The listing builds one solid part. Answer for the finished solid, in the listing's coordinates (mm). Face numbers are marked on the shaded views. A direction names the side the tool comes from. Give positions to 0.01 mm unless a question says otherwise; leave off trailing zeros. Order: outer loops, then holes, each group sorted by start corner. A loop starts at its lowest first (then second) coordinate and runs counter-clockwise, first axis right, second up. Notation, with made-up numbers: (-13, 24) -> (28, 24) arc R22 ccw to (28, 37) -> close; hole circle Ø4 at (57.25, -11). An arc over 180 degrees is marked (long way). Write item = value, one per line. Start each with the question number.
```python
from build123d import *

# Parameters (mm, degrees)
F0_W      = 1219.2
F0_H      = 190.5
F0_W_2    = 1181.1
F0_H_2    = 152.4
F1_DEPTH  = 762
F2_W      = 1219.2
F2_H      = 190.5
F2_W_2    = 1181.1
F2_H_2    = 152.4
F3_DEPTH  = 762
F4_W      = 1219.2
F4_H      = 622.3
F4_W_2    = 1181.1
F4_H_2    = 584.2
F5_DEPTH  = 762
F6_W      = 1219.2
F6_H      = 622.3
F6_W_2    = 1181.1
F6_H_2    = 584.2
F7_DEPTH  = 762
F8_W      = 2438.4
F8_H      = 127
F9_DEPTH  = 6.35
F10_W     = 2438.4
F10_H     = 812.8
F11_DEPTH = 19.05
F12_R     = 38.1
F13_DEPTH = 152.4
F14_W     = 19.05
F14_H     = 152.4
F15_DEPTH = 762
F17_W     = 121.444046
F17_H     = 6.35
F18_DEPTH = 2438.4


with BuildPart() as f1:
    # F0 (on Front) → F1 (new body)
    with BuildSketch(Plane.XZ):
        with Locations((-609.6, 95.25)):
            Rectangle(F0_W, F0_H)
        with Locations((-609.6, 95.25)):
            Rectangle(F0_W_2, F0_H_2, mode=Mode.SUBTRACT)
    extrude(amount=F1_DEPTH)

    # F2 (on Front) → F3 (join)
    with BuildSketch(Plane.XZ):
        with Locations((609.6, 95.25)):
            Rectangle(F2_W, F2_H)
        with Locations((609.6, 95.25)):
            Rectangle(F2_W_2, F2_H_2, mode=Mode.SUBTRACT)
    extrude(amount=F3_DEPTH)

    # F4 (on Front) → F5 (join)
    with BuildSketch(Plane.XZ):
        with Locations((-609.6, -311.15)):
            Rectangle(F4_W, F4_H)
        with Locations((-609.6, -311.15)):
            Rectangle(F4_W_2, F4_H_2, mode=Mode.SUBTRACT)
    extrude(amount=F5_DEPTH)

    # F6 (on Front) → F7 (join)
    with BuildSketch(Plane.XZ):
        with Locations((609.6, -311.15)):
            Rectangle(F6_W, F6_H)
        with Locations((609.6, -311.15)):
            Rectangle(F6_W_2, F6_H_2, mode=Mode.SUBTRACT)
    extrude(amount=F7_DEPTH)

    # F8 (on face) → F9 (cut)
    with BuildSketch(Plane.XY.offset(190.5)):
        with Locations((0, -622.3)):
            Rectangle(F8_W, F8_H)
    extrude(amount=-F9_DEPTH, mode=Mode.SUBTRACT)

    # F10 (on face) → F11 (join)
    with BuildSketch(Plane.XZ.offset(762)):
        with Locations((0, -215.9)):
            Rectangle(F10_W, F10_H)
    extrude(amount=F11_DEPTH)

    # F12 (on face) → F13 (join)
    with BuildSketch(Plane(origin=(0, 0, -622.3), x_dir=(1, 0, 0), z_dir=(0, 0, -1))):
        with Locations((1119.462132, 109.381564)):
            Circle(F12_R)
        with Locations((-1137.543082, 710.901141)):
            Circle(F12_R)
        with Locations((1119.462132, 710.901141)):
            Circle(F12_R)
        with Locations((-1137.543082, 109.381564)):
            Circle(F12_R)
    extrude(amount=F13_DEPTH)

    # F14 (on face) → F15 (join, through all)
    with BuildSketch(Plane(origin=(0, 0, 0), x_dir=(-1, 0, 0), z_dir=(0, 1, 0))):
        with Locations((-609.6, 95.25)):
            Rectangle(F14_W, F14_H)
    extrude(amount=-F15_DEPTH)

    # F16: F1 across plane


with BuildPart() as f1_1:
    add(f1.part)
    add(f1.part.mirror(Plane.YZ))

    # F17 (on face) → F18 (join, through all)
    with BuildSketch(Plane.YZ.offset(1219.2)):
        with Locations((-622.395009, 187.325)):
            Rectangle(F17_W, F17_H)
    extrude(amount=-F18_DEPTH)


solid = f1_1.part
```
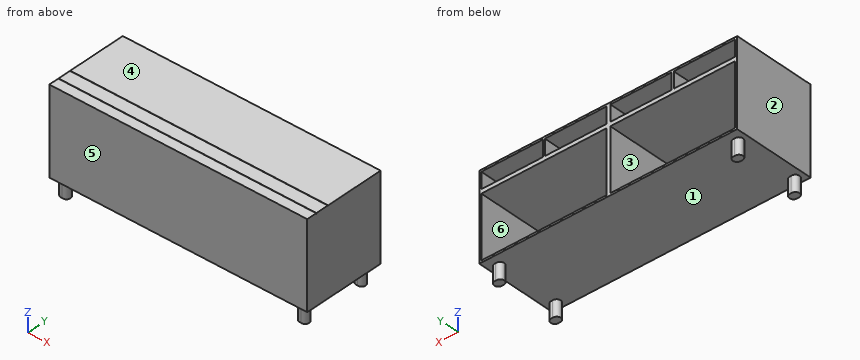
Item 1: A cutting plane is placed at A-A, the plane y = -398. Write down the section's boundary in (x, z) (3 decimals), plus the area to 3 significant figures.
Item 2: The mould has two halves that part along X. Classify the marked faces 1, 2, 3 and 4: +X half, -X half, draft (parallel to the pull), parting line (faces both ways), or undercut.
Item 3: Consider L1, parallel to Z at x = 814, y = -173.5; L2, parallel to X at y = -582, z = -286; L3, parallel to X at y = -662, z = 66.5 (3 decimals). Determine where each line is inside the solid, lowest interval first. Write a range as from..to.
Item 4: A cutting plane is placed at B-B, the plane x = -143. Write down the section's boundary in (y, z).
Item 5: Which of the six approach directions +Z, -Z, +X, -X, +Y, -Y give full straight-line access (tool end or side, diameter ignored) to the marked faces 5 and 6?
Item 6: A cutting plane is placed at C-C, the plane z = -699.5. Write down the section's boundary in (x, y), plus the area to 3 significant figures.
Item 7: A cutting plane is placed at D-D, the plane z = -161. Write down the section's boundary in (x, y).
Check values:
q1.outline = (-1219.2, -622.3) -> (1219.2, -622.3) -> (1219.2, 190.5) -> (-1219.2, 190.5) -> close; hole (-1200.15, -603.25) -> (-19.05, -603.25) -> (-19.05, -19.05) -> (-1200.15, -19.05) -> close; hole (-1200.15, 19.05) -> (-619.125, 19.05) -> (-619.125, 171.45) -> (-1200.15, 171.45) -> close; hole (-600.075, 19.05) -> (-19.05, 19.05) -> (-19.05, 171.45) -> (-600.075, 171.45) -> close; hole (19.05, -603.25) -> (1200.15, -603.25) -> (1200.15, -19.05) -> (19.05, -19.05) -> close; hole (19.05, 19.05) -> (600.075, 19.05) -> (600.075, 171.45) -> (19.05, 171.45) -> close; hole (619.125, 19.05) -> (1200.15, 19.05) -> (1200.15, 171.45) -> (619.125, 171.45) -> close
q1.area = 248,000 mm^2
q2.face_1 = undercut
q2.face_2 = -X half
q2.face_3 = undercut
q2.face_4 = draft
q3.L1 = -622.3..-603.25, -19.05..19.05, 171.45..190.5
q3.L2 = -1219.2..-1200.15, -19.05..19.05, 1200.15..1219.2
q3.L3 = -1219.2..-1200.15, -619.125..-600.075, -19.05..19.05, 600.075..619.125, 1200.15..1219.2
q4.outline = (-781.05, -622.3) -> (0, -622.3) -> (0, -603.25) -> (-762, -603.25) -> (-762, -19.05) -> (0, -19.05) -> (0, 19.05) -> (-762, 19.05) -> (-762, 171.45) -> (0, 171.45) -> (0, 190.5) -> (-558.8, 190.5) -> (-558.8, 184.15) -> (-561.67, 184.15) -> (-561.67, 190.5) -> (-683.12, 190.5) -> (-683.12, 184.15) -> (-685.8, 184.15) -> (-685.8, 190.5) -> (-781.05, 190.5) -> close
q5.face_5 = +Z, -Z, +X, -X, -Y
q5.face_6 = +Y
q6.outline = (-1128.5, -747.91) arc R38.1 ccw (long way) to (-1128.5, -673.89) arc R38.1 ccw (long way) to start; (-1128.5, -146.39) arc R38.1 ccw (long way) to (-1128.5, -72.37) arc R38.1 ccw (long way) to start; (1128.5, -747.91) arc R38.1 ccw (long way) to (1128.5, -673.89) arc R38.1 ccw (long way) to start; (1128.5, -146.39) arc R38.1 ccw (long way) to (1128.5, -72.37) arc R38.1 ccw (long way) to start
q6.area = 23,700 mm^2
q7.outline = (-1219.2, -781.05) -> (1219.2, -781.05) -> (1219.2, 0) -> (1200.15, 0) -> (1200.15, -762) -> (19.05, -762) -> (19.05, 0) -> (-19.05, 0) -> (-19.05, -762) -> (-1200.15, -762) -> (-1200.15, 0) -> (-1219.2, 0) -> close
